Could you check a few things on this model? Use its own coordinates, in mm. A direction names the side the tool comes from. Coordinates: 2 decimals unless noted, no trailing zeros. Order: outer loops, then holes, each group sorted by start corner. A loop starts at its lowest first (then second) coordinate and runs counter-clockwise, first axis right, second up. Notation, with made-up numbers: (30, 66) - (89, 66) arc R18 ccw to (89, 81) - close; hole circle Ø5 at (22, 71.25). An arc over 180 degrees is marked (long way). Answer as a JSON object with one key per item and string values. Group by question number.
(1) Please list where these lines run through material, in increasing order: probe 1 along Z at (x, y) = (0, -7.25); probe 2 along Z at (x, y) = (5, -53); probe 3 along Z at (x, y) = (0, -21).
(2) Imagine slicing it at D-D, the plane z = -4. Write out the boundary of the cut face in (x, y), and give its area (3 significant figures).
(3) Which directions (+Z, -Z, +X, -X, +Y, -Y) give clear straight access to the entire face, cutting with the end or side of a thin tool? Please do faces 4 (the flat face through (0, -27, 0)), 5 (the flat face through (7.5, -64, 40)), 6 (the flat face through (-4, -11, -9)), 7 (the flat face through (0, -35, 16.5)), 8 (the flat face through (0, -51, 13)).
(4) Imagine slicing it at B-B, the plane z = 3. Write out the boundary of the cut face in (x, y).
(5) Will these pins go through, and if not, where does the flat tip stop? P1, Ø4.5, axis at x = 3, y = -32, coming from the -Z side; P2, Ø17, axis at x = 2.5, z = 1, coming from the -Y side; P3, Ø3, axis at x = -8, z = 0.5, coming from the +Y side; P4, Ø6.5, axis at x = 2, z = 2, coming from the +Y side.
(6) Imagine slicing it at A-A, the plane y = -38. Write out the boundary of the cut face in (x, z).
(7) Imagine slicing it at C-C, the plane y = -8.5. Write out the boundary of the cut face in (x, z), and give its area (3 significant figures).
(8) We'd pull the mould along Z, two halves only. Please class faces 1 (the cylindrical face through (4.619, -29.415, 13.38)), 2 (the flat face through (-7.5, -64, 40)), 3 (the flat face through (11.2, -50.9, -6.6)): pulls with the +Z half, pulls with the -Z half, needs draft (parallel to the pull), parting line crosses it, or undercut.
from build123d import *

# Parameters (mm, degrees)
F0_R     = 9.3155
F1_DEPTH = 11
F2_R     = 12
F2_R_2   = 10.5
F3_DEPTH = 34.5
F4_R     = 9.3155
F5_DEPTH = 11
F6_R     = 5
F7_DEPTH = 18
F9_DEPTH = 7.5


with BuildPart() as f1:
    # F0 (on Front) → F1 (new body)
    with BuildSketch(Plane.XZ):
        Polygon((-7.5055534995, 13), (-15.0111069989, 0), (-7.5055534995, -13), (7.5055534995, -13), (15.0111069989, 0), (7.5055534995, 13), align=None)
        Circle(F0_R, mode=Mode.SUBTRACT)
    extrude(amount=F1_DEPTH)

    # F2 (on face) → F3 (join)
    with BuildSketch(Plane.XZ.offset(11)):
        Circle(F2_R)
        Circle(F2_R_2, mode=Mode.SUBTRACT)
    extrude(amount=F3_DEPTH)

    # F4 (on face) → F5 (join)
    with BuildSketch(Plane.XZ.offset(45.5)):
        Polygon((-7.5055534995, 13), (-15.0111069989, 0), (-7.5055534995, -13), (7.5055534995, -13), (15.0111069989, 0), (7.5055534995, 13), align=None)
        Circle(F4_R, mode=Mode.SUBTRACT)
    extrude(amount=F5_DEPTH)

    # F6 (on Top) → F7 (join)
    with BuildSketch(Plane.XY):
        with Locations((0, -27.5)):
            Circle(F6_R)
    extrude(amount=F7_DEPTH)

    # F8 (on Right) → F9 (join, symmetric)
    with BuildSketch(Plane.YZ):
        Polygon((-20, 15), (-20, 16.5), (-44.8413931031, 16.5), (-49.9539528364, 40.5), (-114.5, 40.5), (-114.5, 39), (-52.2972028911, 39), (-46.7586030031, 15), align=None)
    extrude(amount=F9_DEPTH, both=True)


solid = f1.part
Result set:
{
 "1": {"probe 1": "z = -13 to -9.32, 9.32 to 13", "probe 2": "z = -13 to -7.86, 7.86 to 13, 39 to 40.5", "probe 3": "z = -12 to -10.5, 10.5 to 12, 15 to 16.5"},
 "2": {"outline": "(-12.7, -56.5) - (-8.41, -56.5) - (-8.41, -45.5) - (-9.71, -45.5) - (-9.71, -11) - (-8.41, -11) - (-8.41, 0) - (-12.7, 0) - (-12.7, -11) - (-11.31, -11) - (-11.31, -45.5) - (-12.7, -45.5) - close; (8.41, -56.5) - (12.7, -56.5) - (12.7, -45.5) - (11.31, -45.5) - (11.31, -11) - (12.7, -11) - (12.7, 0) - (8.41, 0) - (8.41, -11) - (9.71, -11) - (9.71, -45.5) - (8.41, -45.5) - close", "area": "299 mm^2"},
 "3": {"face 4": "+Y, -Y", "face 5": "+Z, +X, +Y, -Y", "face 6": "none", "face 7": "+Z", "face 8": "+X, -X, -Y"},
 "4": {"outline": "(-13.28, -56.5) - (-8.82, -56.5) - (-8.82, -45.5) - (-10.06, -45.5) - (-10.06, -11) - (-8.82, -11) - (-8.82, 0) - (-13.28, 0) - (-13.28, -11) - (-11.62, -11) - (-11.62, -45.5) - (-13.28, -45.5) - close; circle Ø10 at (0, -27.5); (8.82, -56.5) - (13.28, -56.5) - (13.28, -45.5) - (11.62, -45.5) - (11.62, -11) - (13.28, -11) - (13.28, 0) - (8.82, 0) - (8.82, -11) - (10.06, -11) - (10.06, -45.5) - (8.82, -45.5) - close"},
 "5": {"P1": "stops at z = -11.98", "P2": "stops at y = -56.5", "P3": "stops at y = 0", "P4": "stops at y = -22.5"},
 "6": {"outline": "circle Ø24 at (0, 0); (-7.5, 15) - (7.5, 15) - (7.5, 16.5) - (-7.5, 16.5) - close; hole circle Ø21 at (0, 0)"},
 "7": {"outline": "(-15.01, 0) - (-7.51, -13) - (7.51, -13) - (15.01, 0) - (7.51, 13) - (-7.51, 13) - close; hole circle Ø18.63 at (0, 0)", "area": "313 mm^2"},
 "8": {"face 1": "undercut", "face 2": "needs draft", "face 3": "pulls with the -Z half"}
}
